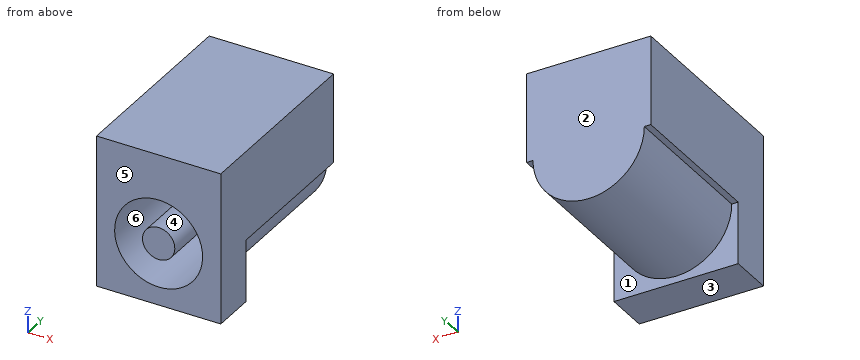
```python
from build123d import *

# Parameters (mm, degrees)
SKETCH1_W           = 8.7884
SKETCH1_H           = 10.7188
BOSS_EXTRUDE1_DEPTH = 13.589
CUT_EXTRUDE1_DEPTH  = 10.541
SKETCH3_R           = 3.1115
SKETCH3_R_2         = 1.143
CUT_EXTRUDE2_DEPTH  = 11.049


with BuildPart() as part:
    # Sketch1 → Boss-Extrude1 (new body)
    with BuildSketch(Plane(origin=(0, 0, 0), x_dir=(1, 0, 0), z_dir=(0, 1, 0))):
        with Locations((4.3942, 5.3594)):
            Rectangle(SKETCH1_W, SKETCH1_H)
    extrude(amount=BOSS_EXTRUDE1_DEPTH)

    # Sketch2 → Cut-Extrude1 (cut)
    with BuildSketch(Plane(origin=(0, 13.589, 0), x_dir=(1, 0, 0), z_dir=(0, 1, 0))):
        with BuildLine():
            Line((0.4572, 6.3246), (0, 6.3246))
            Line((0, 6.3246), (0, 10.7188))
            Line((0, 10.7188), (8.7884, 10.7188))
            Line((8.7884, 10.7188), (8.7884, 6.3246))
            Line((8.7884, 6.3246), (8.3312, 6.3246))
            ThreePointArc((8.3312, 6.3246), (4.3942, 10.2616), (0.4572, 6.3246))
        make_face()
    extrude(amount=-CUT_EXTRUDE1_DEPTH, mode=Mode.SUBTRACT)

    # Sketch3 → Cut-Extrude2 (cut)
    with BuildSketch(Plane.XZ):
        with Locations(Location((4.3942, -6.3246, 0), (0, 0, 270))):
            Circle(SKETCH3_R)
        with Locations(Location((4.3942, -6.3246, 0), (0, 0, 270))):
            Circle(SKETCH3_R_2, mode=Mode.SUBTRACT)
    extrude(amount=-CUT_EXTRUDE2_DEPTH, mode=Mode.SUBTRACT)


solid = part.part
```
The listing builds one solid part. Answer for the finished solid, in the listing's coordinates (mm). Face numbers are marked on the shaded views. A direction names the side the tool comes from. Give positions to 0.01 mm unless a question says otherwise; leave off trailing zeros. Order: outer loops, then holes, each group sorted by start corner. A loop starts at its lowest first (then second) coordinate and runs counter-clockwise, first axis right, second up. Notation, with made-up numbers: (-18.5, 24.5) - (12.5, 24.5) arc R27 ccw to (12.5, 57.5) - close; hole circle Ø7 at (-2, 81). An arc over 180 degrees is marked (long way). Use one line per item in the form item = value. Start each with the question number.
(1) Consider line 1 (Z direction, x = 5, y = 1); line 2 (Z direction, x = 3.75, y = 8.5); line 3 (X direction, y = 1.5, z = -6.5). Determine where each line is inside the solid, lowest interval first. Write a range as from..to.
(2) Flat-ended cylindrical pins translate along their axes: pin 1 Ø1.5 at (x, y) = (3.5, 9.5) entering from -Z; pin 2 Ø1 at (x, y) = (3, 6.5) entering from -Z. Find the tip coordinate at first contact, or state that the pin passes through.
(3) A cutting plane is placed at C-C, the plane z = -6.5. Write down the section's boundary in (x, y).
(4) The mould has two halves that part along Z. Classify the marked faces 3, 4, 5 and 6: released by +Z, released by -Z, zero draft, split by the parting line, or undercut.
(5) A cutting plane is placed at B-B, the plane x = 5.75. Write down the section's boundary in (y, z), then the cut area to 3 significant figures.
(6) A cutting plane is placed at D-D, the plane y = 2.5. Write down the section's boundary in (x, z).
(7) For the marked faces 1 and 2, determine the directions among +Z, -Z, +X, -X, +Y, -Y from which every point of the face is accessible in a straight line to the end or side of a thin tool.
Ans:
q1.line_1 = -10.72..-9.38, -7.29..-5.36, -3.27..0
q1.line_2 = -10.21..-9.37, -7.27..-5.38, -3.28..0
q1.line_3 = 0..1.29, 3.26..5.52, 7.5..8.79
q2.pin_1 = -10.26
q2.pin_2 = -10.16
q3.outline = (0, 0) - (1.29, 0) - (1.29, 11.05) - (3.26, 11.05) - (3.26, 0) - (5.52, 0) - (5.52, 11.05) - (7.5, 11.05) - (7.5, 0) - (8.79, 0) - (8.79, 3.05) - (8.33, 3.05) - (8.33, 13.59) - (0.46, 13.59) - (0.46, 3.05) - (0, 3.05) - close
q4.face_3 = released by -Z
q4.face_4 = undercut
q4.face_5 = zero draft
q4.face_6 = undercut
q5.outline = (0, -10.72) - (3.05, -10.72) - (3.05, -10.02) - (13.59, -10.02) - (13.59, 0) - (0, 0) - (0, -3.52) - (11.05, -3.52) - (11.05, -9.13) - (0, -9.13) - close
q5.area = 76.4 mm^2
q6.outline = (0, -10.72) - (8.79, -10.72) - (8.79, 0) - (0, 0) - close; circle Ø2.29 at (4.39, -6.32); hole circle Ø6.22 at (4.39, -6.32)
q7.face_1 = -Z, +Y
q7.face_2 = +Z, -Z, +X, -X, +Y
